from build123d import *

# Parameters (mm, degrees)
SKETCH_2_R          = 1.1
SKETCH_2_R_2        = 1
SKETCH_2_R_3        = 1.7
EXTRUDE_1_DEPTH     = 2
SKETCH_3_W          = 10.4
SKETCH_3_H          = 12.4
EXTRUDE_2_DEPTH     = 9.5
SKETCH_4_W          = 10.4
SKETCH_4_H          = 12.4
CUT_EXTRUDE_1_DEPTH = 0.5
SKETCH_5_R          = 2.25
CUT_EXTRUDE_2_DEPTH = 0.9
CHAMFER_1_SIZE      = 0.5


with BuildPart() as part:
    # Эскиз2 → Бобышка-Вытянуть1 (new body)
    with BuildSketch(Plane.XY):
        with BuildLine():
            Line((6.21, 6.514284305), (11.449, 1.519999671))
            ThreePointArc((11.449, 1.519999671), (12.1, 0), (11.449, -1.519999671))
            Line((11.449, -1.519999671), (6.21, -6.514284305))
            ThreePointArc((6.21, -6.514284305), (0, -9), (-6.21, -6.514284305))
            Line((-6.21, -6.514284305), (-11.449, -1.519999671))
            ThreePointArc((-11.449, -1.519999671), (-12.1, 0), (-11.449, 1.519999671))
            Line((-11.449, 1.519999671), (-6.21, 6.514284305))
            ThreePointArc((-6.21, 6.514284305), (0, 9), (6.21, 6.514284305))
        make_face()
        with Locations((10, 0)):
            Circle(SKETCH_2_R, mode=Mode.SUBTRACT)
        with Locations((-10, 0)):
            Circle(SKETCH_2_R, mode=Mode.SUBTRACT)
        with Locations((0, 4.5)):
            Circle(SKETCH_2_R_2, mode=Mode.SUBTRACT)
        with Locations(Location((0, -4.5, 0), (0, 0, 180))):
            Circle(SKETCH_2_R_2, mode=Mode.SUBTRACT)
        Circle(SKETCH_2_R_3, mode=Mode.SUBTRACT)
    extrude(amount=EXTRUDE_1_DEPTH)

    # Эскиз3 → Бобышка-Вытянуть2 (add)
    with BuildSketch(Plane.XY.offset(2)):
        with BuildLine():
            Line((6.21, 6.514284305), (6.21, -6.514284305))
            ThreePointArc((6.21, -6.514284305), (0, -9), (-6.21, -6.514284305))
            Line((-6.21, -6.514284305), (-6.21, 6.514284305))
            ThreePointArc((-6.21, 6.514284305), (0, 9), (6.21, 6.514284305))
        make_face()
        Rectangle(SKETCH_3_W, SKETCH_3_H, mode=Mode.SUBTRACT)
    extrude(amount=EXTRUDE_2_DEPTH)

    # Эскиз4 → Вырез-Вытянуть1 (cut)
    with BuildSketch(Plane.XY.offset(2)):
        Rectangle(SKETCH_4_W, SKETCH_4_H)
    extrude(amount=-CUT_EXTRUDE_1_DEPTH, mode=Mode.SUBTRACT)

    # Эскиз5 → Вырез-Вытянуть2 (cut)
    with BuildSketch(Plane.XY.offset(1.5)):
        Circle(SKETCH_5_R)
    extrude(amount=-CUT_EXTRUDE_2_DEPTH, mode=Mode.SUBTRACT)

    # Фаска1
    chamfer_1_edges = [part.edges().sort_by_distance(p)[0] for p in [
        (-8.8295, 4.017141988, 0),
        (0, 9, 0),
        (8.9, 0, 0),
        (-1, 4.5, 0),
        (1, -4.5, 0),
        (-1.7, 0, 0),
        (-11.1, 0, 0),
        (8.8295, 4.017141988, 0),
        (12.1, 0, 0),
        (8.8295, -4.017141988, 0),
        (0, -9, 0),
        (-8.8295, -4.017141988, 0),
        (-12.1, 0, 0),
    ]]
    chamfer(chamfer_1_edges, length=CHAMFER_1_SIZE - 0.0001)  # a hair under: the kernel refuses the full size


solid = part.part
Verification items for the finished model (mm, model axes). A direction names the side the tool comes from. Give positions to 0.01 mm unless a question says otherwise; leave off trailing zeros. Loops run counter-clockwise (first coordinate to the right, second up) from the corner with the lowest first, then second, coordinate; pieces in that order, holes last. Notation, with made-up numbers: (-10, -5) - (43, -5) arc R21 ccw to (43, 31) - close; hole circle Ø4 at (29.25, 30.25). An arc over 180 degrees is marked (long way). Write item = value, one per line. Start each with the question number.
Q1. Depth check by flat-ended pin: P1, Ø2, axis at x = -1, z = 10, coming from the +Y side; P2, Ø4, axis at x = -6.5, z = 3, coming from the +Y side; P3, Ø2.5, axis at x = 0, y = -4.5, coming from the -Z side; P4, Ø3.5, axis at x = 0, y = 0, coming from the -Z side. Enter the tip coordinate at first touch or a pass-through.
Q2. Cross-section at B-B, the plane x = 0. State how many separate pieces and enclosed holes the cut face has, and give its area (3 significant figures).
Q3. Tool access check on faces 4 (the face through (8.62, 3.87, 0.25)), 5 (the face through (-0.29, 2.23, 1.06)), 6 (the face through (6.21, 0, 7)). Record the directions out of +Z, -Z, +X, -X, +Y, -Y that give a thin tool (end or side, any length) a straight path to the whole face; none if there is none.
Q4. Cross-section at C-C, the plane y = 4.5. Enter the section's corners in (x, z).
Q5. Cross-section at D-D, the plane x = -10. Enter the section's corners in (y, z).
Q6. Thickness scan on line 1 (Y direction, x = 0, z = 1.25); line 2 (X direction, y = -3, z = 2.25); line 3 (Z direction, x = 2.5, y = 5). Record the ranges inside material, lowest first.
Q7. Cross-section at A-A, the plane z = 3.75. Enter the section's corners in (x, y).
Q8. Mould release check, pull along X, two halves, no side actions. Record for faces 1 (the face through (0.13, -5.49, 0.99)), 2 (the face through (0, -9, 6)), 3 (the face through (-2.4, 0.1, 0)): released by +X, released by -X, zero draft, split by the parting line, or undercut.
Answer key:
q1.P1 = 9
q1.P2 = 7.79
q1.P3 = 0.25
q1.P4 = 0.45
q2.separate_pieces = 4
q2.enclosed_holes = 0
q2.area = 69.9 mm^2
q3.face_4 = -Z, +X, +Y
q3.face_5 = +Z
q3.face_6 = +Z, +X, +Y, -Y
q4.outline = (-8.32, 0.5) - (-7.6, 0) - (-1.5, 0) - (-1, 0.5) - (-1, 1.5) - (-5.2, 1.5) - (-5.2, 11.5) - (-6.21, 11.5) - (-6.21, 2) - (-8.32, 2) - close; (1, 0.5) - (1.5, 0) - (7.6, 0) - (8.32, 0.5) - (8.32, 2) - (6.21, 2) - (6.21, 11.5) - (5.2, 11.5) - (5.2, 1.5) - (1, 1.5) - close
q5.outline = (-2.9, 0.5) - (-2.21, 0) - (-1.6, 0) - (-1.1, 0.5) - (-1.1, 2) - (-2.9, 2) - close; (1.1, 0.5) - (1.6, 0) - (2.21, 0) - (2.9, 0.5) - (2.9, 2) - (1.1, 2) - close
q6.line_1 = -9 to -5.5, -3.5 to -2.25, 2.25 to 3.5, 5.5 to 9
q6.line_2 = -6.21 to -5.2, 5.2 to 6.21
q6.line_3 = 0 to 1.5
q7.outline = (-6.21, -6.51) arc R9 ccw to (6.21, -6.51) - (6.21, 6.51) arc R9 ccw to (-6.21, 6.51) - close; hole (-5.2, -6.2) - (5.2, -6.2) - (5.2, 6.2) - (-5.2, 6.2) - close
q8.face_1 = undercut
q8.face_2 = split by the parting line
q8.face_3 = zero draft
